Autodesk Inventor part; units mm, degrees
ref_plane "YZ Plane" through (0, 0, 0) normal (1, 0, 0) x (0, 1, 0)
ref_plane "XZ Plane" through (0, 0, 0) normal (0, 1, 0) x (-1, 0, 0)
ref_plane "XY Plane" through (0, 0, 0) normal (0, 0, 1) x (1, 0, 0)
sketch "Sketch1" plane through (0, 0, 0) normal (0, 0, 1) x (1, 0, 0)
  line L0 (-6.0434, 5.1689) -> (-6.0434, -5.8039) construction
  line L1 (-6.0434, -5.8039) -> (6.0216, -5.8039) construction
  line L2 (6.0216, -5.8039) -> (6.0216, 5.1689) construction
  line L3 (6.0216, 5.1689) -> (-6.0434, 5.1689) construction
  line L4 (-4.2654, -4.0259) -> (4.2436, -4.0259) construction
  line L5 (-4.2654, 2.4003) -> (-4.2654, -4.0259) construction
  line L6 (-2.7795, 4.0259) -> (-4.2654, 2.4003) construction
  line L7 (2.7577, 4.0259) -> (-2.7795, 4.0259) construction
  line L8 (4.2436, 2.4003) -> (2.7577, 4.0259) construction
  line L9 (4.2436, -4.0259) -> (4.2436, 2.4003) construction
  line L10 (-4.2654, -4.0259) -> (4.2436, -4.0259) construction
  line L11 (4.2436, -4.0259) -> (4.2436, 2.4003) construction
  line L12 (4.2436, 2.4003) -> (2.7577, 4.0259) construction
  line L13 (2.7577, 4.0259) -> (-2.7795, 4.0259) construction
  line L14 (-2.7795, 4.0259) -> (-4.2654, 2.4003) construction
  line L15 (-4.2654, 2.4003) -> (-4.2654, -4.0259) construction
  line L16 (1.9887, -1.7399) -> (2.7831, -1.7399) construction
  line L17 (1.9887, -1.8669) -> (1.9887, -1.7399) construction
  line L18 (1.9887, -1.8669) -> (1.0213, -1.8669) construction
  line L19 (1.0213, -1.8669) -> (1.0213, -1.7399) construction
  line L20 (-1.0213, -1.7399) -> (1.0213, -1.7399) construction
  line L21 (-1.0213, -1.8669) -> (-1.0213, -1.7399) construction
  line L22 (-1.0213, -1.8669) -> (-1.9887, -1.8669) construction
  line L23 (-1.9887, -1.8669) -> (-1.9887, -1.7399) construction
  line L24 (-2.8049, -1.7399) -> (-1.9887, -1.7399) construction
  line L25 (-2.8049, 1.7399) -> (-2.8049, -1.7399) construction
  line L26 (-1.9887, 1.7399) -> (-2.8049, 1.7399) construction
  line L27 (-1.9887, 1.8669) -> (-1.9887, 1.7399) construction
  line L28 (-1.0213, 1.8669) -> (-1.9887, 1.8669) construction
  line L29 (-1.0213, 1.8669) -> (-1.0213, 1.7399) construction
  line L30 (1.0213, 1.7399) -> (-1.0213, 1.7399) construction
  line L31 (1.0213, 1.8669) -> (1.0213, 1.7399) construction
  line L32 (1.9887, 1.8669) -> (1.0213, 1.8669) construction
  line L33 (1.9887, 1.8669) -> (1.9887, 1.7399) construction
  line L34 (2.7831, 1.7399) -> (1.9887, 1.7399) construction
  line L35 (2.7831, -1.7399) -> (2.7831, 1.7399) construction
  line L36 (2.1481, -1.1049) -> (2.1481, 1.1049) construction
  line L37 (2.1481, 1.1049) -> (-2.1699, 1.1049) construction
  line L38 (-2.1699, 1.1049) -> (-2.1699, -1.1049) construction
  line L39 (-2.1699, -1.1049) -> (2.1481, -1.1049) construction
  line L40 (-2.8049, 0) -> (2.7831, 0) construction
  line L41 (0, 1.7399) -> (0, -1.7399) construction
  point P0 (0, 0)
  point P1 (0, 0)
sketch "Sketch2" plane through (0, 0, 0) normal (0, 0, 1) x (1, 0, 0)
  line L0 (6.0216, 5.1689) -> (-6.0434, 5.1689)
  line L1 (-6.0434, 5.1689) -> (-6.0434, -5.8039)
  line L2 (-6.0434, -5.8039) -> (6.0216, -5.8039)
  line L3 (6.0216, -5.8039) -> (6.0216, 5.1689)
  line L4 (-4.2654, -4.0259) -> (4.2436, -4.0259)
  line L5 (4.2436, -4.0259) -> (4.2436, 2.4003)
  line L6 (4.2436, 2.4003) -> (2.7577, 4.0259)
  line L7 (2.7577, 4.0259) -> (-2.7795, 4.0259)
  line L8 (-2.7795, 4.0259) -> (-4.2654, 2.4003)
  line L9 (-4.2654, 2.4003) -> (-4.2654, -4.0259)
  point P0 (0, 0)
extrude "Extrusion1" add sketch "Sketch2" along normal blind 9.11
sketch "Sketch3" plane through (0, 0, 0) normal (0, 0, -1) x (-1, 0, 0)
  line L0 (-6.0216, 5.1689) -> (6.0434, 5.1689)
  line L1 (6.0434, 5.1689) -> (6.0434, -5.8039)
  line L2 (6.0434, -5.8039) -> (-6.0216, -5.8039)
  line L3 (-6.0216, -5.8039) -> (-6.0216, 5.1689)
  point P0 (0, 0)
extrude "Extrusion2" add sketch "Sketch3" along normal blind 1
sketch "Sketch4" plane through (0, 0, 0) normal (0, 0, 1) x (1, 0, 0)
  line L0 (-1.9887, 1.7399) -> (-2.8049, 1.7399) construction
  line L1 (-2.8049, 1.7399) -> (-2.8049, -1.7399) construction
  line L2 (1.9887, -1.7399) -> (2.7831, -1.7399) construction
  line L3 (2.7831, -1.7399) -> (2.7831, 1.7399) construction
  line L4 (-2.8049, 1.7399) -> (2.7831, 1.7399)
  line L5 (2.7831, 1.7399) -> (2.7831, -1.7399)
  line L6 (2.7831, -1.7399) -> (-2.8049, -1.7399)
  line L7 (-2.8049, -1.7399) -> (-2.8049, 1.7399)
  point P0 (0, 0)
extrude "Extrusion3" add sketch "Sketch4" along normal blind 8.11
sketch "Sketch5" plane through (0, 0, 8.11) normal (0, 0, 1) x (1, 0, 0)
  line L0 (2.7831, 1.7399) -> (-2.8049, 1.7399)
  line L1 (-2.8049, 1.7399) -> (-2.8049, -1.7399)
  line L2 (-2.8049, -1.7399) -> (2.7831, -1.7399)
  line L3 (2.7831, -1.7399) -> (2.7831, 1.7399)
  point P0 (0, 0)
extrude "Extrusion4" add sketch "Sketch5" along normal blind 1 draft -25
sketch "Sketch6" plane through (0, 0, 0) normal (0, 0, 1) x (1, 0, 0)
  line L0 (-1.0213, 1.8669) -> (-1.9887, 1.8669) construction
  line L1 (1.9887, 1.8669) -> (1.0213, 1.8669) construction
  line L2 (1.9887, -1.8669) -> (1.0213, -1.8669) construction
  line L3 (-1.0213, -1.8669) -> (-1.9887, -1.8669) construction
  line L4 (-1.9887, 1.8669) -> (-1.0213, 1.8669)
  line L5 (-1.0213, 1.8669) -> (-1.0213, 1.7421)
  line L6 (-1.0213, 1.7421) -> (-1.9887, 1.7421)
  line L7 (-1.9887, 1.7421) -> (-1.9887, 1.8669)
  line L8 (1.0213, 1.8669) -> (1.9887, 1.8669)
  line L9 (1.9887, 1.8669) -> (1.9887, 1.7421)
  line L10 (1.9887, 1.7421) -> (1.0213, 1.7421)
  line L11 (1.0213, 1.7421) -> (1.0213, 1.8669)
  line L12 (-1.9887, -1.8669) -> (-1.0213, -1.8669)
  line L13 (-1.0213, -1.8669) -> (-1.0213, -1.7274)
  line L14 (-1.0213, -1.7274) -> (-1.9887, -1.7274)
  line L15 (-1.9887, -1.7274) -> (-1.9887, -1.8669)
  line L16 (1.0213, -1.8669) -> (1.9887, -1.8669)
  line L17 (1.9887, -1.8669) -> (1.9887, -1.7274)
  line L18 (1.9887, -1.7274) -> (1.0213, -1.7274)
  line L19 (1.0213, -1.7274) -> (1.0213, -1.8669)
  point P0 (0, 0)
extrude "Extrusion5" add sketch "Sketch6" along normal blind 6.84
fillet "Fillet1" radius 0.3 4 edges at (6.0216, 5.1689, 4.055) (6.0216, -5.8039, 4.055) (-6.0434, -5.8039, 4.055) (-6.0434, 5.1689, 4.055)
properties part number "USB B Female Port" material "Steel, Mild"
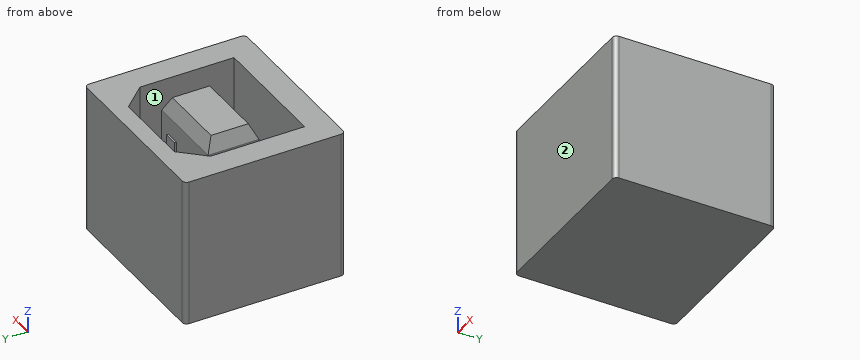
Part model, mm, in its own coordinate system. Face numbers are marked on the shaded views. A direction names the side the tool comes from. Coordinates: 2 decimals unless noted, no trailing zeros. Write each loop counter-clockwise with the first axis right and the second up, starting at its lowest first coordinate (ties: lowest second). Pieces come first, ordered by that corner, then holes. Notation, with made-up numbers: M -26,34 L 2,34 A28 ccw 2,63 Z; hole C -10,-16 d4. An arc over 180 degrees is marked long. Return JSON: item names as keys, results as strings.
1. Saw through at D-D, the plane y = -0.5. Write the cut outline in (x, z), then the cut area to 3 significant figures.
Determined:
{"outline": "M -6.04,-1 L 6.02,-1 L 6.02,9.11 L 4.24,9.11 L 4.24,0 L 2.78,0 L 2.78,8.11 L 2.32,9.11 L -2.34,9.11 L -2.8,8.11 L -2.8,0 L -4.27,0 L -4.27,9.11 L -6.04,9.11 Z", "area": "94.9 mm²"}
2. Saw through at B-B, the plane z = 7. Write the cut outline in (x, y), then the cut area to 3 significant figures.
Determined:
{"outline": "M -6.04,-5.5 A0.3 ccw -5.74,-5.8 L 5.72,-5.8 A0.3 ccw 6.02,-5.5 L 6.02,4.87 A0.3 ccw 5.72,5.17 L -5.74,5.17 A0.3 ccw -6.04,4.87 Z; M -2.8,-1.74 L 2.78,-1.74 L 2.78,1.74 L -2.8,1.74 Z; hole M -4.27,-4.03 L 4.24,-4.03 L 4.24,2.4 L 2.76,4.03 L -2.78,4.03 L -4.27,2.4 Z", "area": "85.7 mm²"}
3. 3-axis set-ups, long thin cutter, end or side, ignore diameter. For the marked faces 1 and 2: which of +Z, -Z, +X, -X, +Y, -Y reach the whole face in a straight line?
Determined:
{"face 1": "+Z", "face 2": "+Z, -Z, +X, -X, -Y"}
4. Saw through at A-A, the plane z = 3.5. Count the separate pieces of the cut face and the enclosed holes in it, then the cut area to 3 significant figures.
Determined:
{"separate pieces": "4", "enclosed holes": "1", "area": "86.1 mm²"}
5. Saw through at C-C, the plane y = -2.75. Write the cut outline in (x, z).
Determined:
{"outline": "M -6.04,-1 L 6.02,-1 L 6.02,9.11 L 4.24,9.11 L 4.24,0 L -4.27,0 L -4.27,9.11 L -6.04,9.11 Z"}
6. Probe L1, parallel to X at y = 1.25, z = 1.75; L2, parallel to Y at x = 2.5, z = 8; L3, parallel to X at y = 2.25, z = 6. List the from-to ranges inside material, lowest first.
Determined:
{"L1": "-6.04 to -4.27, -2.8 to 2.78, 4.24 to 6.02", "L2": "-5.8 to -4.03, -1.74 to 1.74, 4.03 to 5.17", "L3": "-6.04 to -4.27, 4.24 to 6.02"}
